Model file for the job. Use its own axes, mm. A direction names the side the tool comes from. Round coordinates to 2 decimals unless told otherwise and drop trailing zeros. Loops run counter-clockwise (first coordinate to the right, second up) from the corner with the lowest first, then second, coordinate; pieces in that order, holes last. Notation, with made-up numbers: (83, -5) -> (100, -5) arc R8 cw to (100, 10) -> close; hole circle Ø3 at (4, 59.25). An arc over 180 degrees is marked (long way). Use a Markdown table: item, result.
from build123d import *

# Parameters (mm, degrees)
SKETCH_R          = 1.5
PAD_DEPTH         = 8
SKETCH001_W       = 18.9
SKETCH001_H       = 25.2
POCKET_DEPTH      = 0.8
SKETCH002_W       = 15
SKETCH002_H       = 2.5
SKETCH002_W_2     = 10.4
POCKET001_DEPTH   = 3
SKETCH003_W       = 6
SKETCH003_H       = 30
PAD001_DEPTH      = 9
SKETCH004_W       = 19.2
SKETCH004_H       = 2
POCKET002_DEPTH   = 2
POCKET003_DEPTH   = 3
PAD002_DEPTH      = 3
PAD002_DEPTH_BACK = 3
PAD003_DEPTH      = 1
CHAMFER_SIZE      = 0.95


with BuildPart() as part:
    # Sketch → Pad (new body)
    with BuildSketch(Plane.XY):
        Polygon((-20.1, 15), (11.9, 15), (30, 3.75), (30, -3.75), (11.9, -15), (-20.1, -15), align=None)
        with Locations((-6.25, 0)):
            Circle(SKETCH_R, mode=Mode.SUBTRACT)
    extrude(amount=-PAD_DEPTH)

    # Sketch001 → Pocket (cut)
    with BuildSketch(Plane.XY):
        Rectangle(SKETCH001_W, SKETCH001_H)
    extrude(amount=-POCKET_DEPTH, mode=Mode.SUBTRACT)

    # Sketch002 (on Face33 of Pad003) → Pocket001 (cut)
    with BuildSketch(Plane.XY.offset(-0.8)):
        with Locations((-0.534042, 8.083783)):
            Rectangle(SKETCH002_W, SKETCH002_H)
        with Locations((2.090713, -8.153236)):
            Rectangle(SKETCH002_W_2, SKETCH002_H)
    extrude(amount=-POCKET001_DEPTH, mode=Mode.SUBTRACT)

    # Sketch003 (on Face4 of Pocket001) → Pad001 (join)
    with BuildSketch(Plane.XY):
        with Locations((-17.1, 0)):
            Rectangle(SKETCH003_W, SKETCH003_H)
    extrude(amount=PAD001_DEPTH)

    # Sketch004 (on Face10 of Pad001) → Pocket002 (cut)
    with BuildSketch(Plane.YZ.offset(-14.1)):
        with Locations((0, 6.14)):
            Rectangle(SKETCH004_W, SKETCH004_H)
    extrude(amount=-POCKET002_DEPTH, mode=Mode.SUBTRACT)

    # Sketch005 → Pocket003 (cut)
    with BuildSketch(Plane(origin=(0, 0, -8), x_dir=(1, 0, 0), z_dir=(0, 0, -1))):
        Polygon((-4.633419, 2.8), (-7.866581, 2.8), (-9.483162, 0), (-7.866581, -2.8), (-4.633419, -2.8), (-3.016838, 0), align=None)
    extrude(amount=-POCKET003_DEPTH, mode=Mode.SUBTRACT)

    # Sketch006 → Pad002 (join, two sides)
    with BuildSketch(Plane.XZ) as pad002_sk:
        Polygon((13.9, 0), (20.9, 5.25), (26.9, 5.25), (26.9, 0), align=None)
    extrude(amount=PAD002_DEPTH)
    extrude(pad002_sk.sketch, amount=-PAD002_DEPTH_BACK)

    # Sketch007 (on Face32 of Pad002) → Pad003 (join)
    with BuildSketch(Plane.XY.offset(5.25)):
        with BuildLine():
            ThreePointArc((24, -1.925), (25.925, 0), (24, 1.925))
            Line((24, 1.925), (23, 1.925))
            Line((23, 1.925), (23, -1.925))
            Line((23, -1.925), (24, -1.925))
        make_face()
    extrude(amount=PAD003_DEPTH)

    # Chamfer
    chamfer_edges = [part.edges().sort_by_distance(p)[0] for p in [
        (23, 0, 6.25),
        (23, -1.925, 5.75),
        (23, 1.925, 5.75),
    ]]
    chamfer(chamfer_edges, length=CHAMFER_SIZE)


solid = part.part
Q1. Band-saw the part on D-D, the plane z = -1.5. Give the cut face in (x, y), plus the area to 3 significant figures.
Results list:
| item | result |
|---|---|
| outline | (-20.1, -15) -> (11.9, -15) -> (30, -3.75) -> (30, 3.75) -> (11.9, 15) -> (-20.1, 15) -> close; hole (-8.03, 6.83) -> (6.97, 6.83) -> (6.97, 9.33) -> (-8.03, 9.33) -> close; hole circle Ø3 at (-6.25, 0); hole (-3.11, -9.4) -> (7.29, -9.4) -> (7.29, -6.9) -> (-3.11, -6.9) -> close |
| area | 1,230 mm² |
Q2. Band-saw the part on C-C, the plane z = 3. Give the cut face in (x, y).
Results list:
| item | result |
|---|---|
| outline | (-20.1, -15) -> (-14.1, -15) -> (-14.1, 15) -> (-20.1, 15) -> close; (17.9, -3) -> (26.9, -3) -> (26.9, 3) -> (17.9, 3) -> close |
Q3. Band-saw the part on A-A, the plane x = -6.25. Give the cut face in (y, z).
Results list:
| item | result |
|---|---|
| outline | (-15, -8) -> (-2.8, -8) -> (-2.8, -5) -> (-1.5, -5) -> (-1.5, -0.8) -> (-12.6, -0.8) -> (-12.6, 0) -> (-15, 0) -> close; (1.5, -5) -> (2.8, -5) -> (2.8, -8) -> (15, -8) -> (15, 0) -> (12.6, 0) -> (12.6, -0.8) -> (9.33, -0.8) -> (9.33, -3.8) -> (6.83, -3.8) -> (6.83, -0.8) -> (1.5, -0.8) -> close |
Q4. Pull direction Y, two halves, no side cores. Call faces 5 (the face through (20.823, 9.454, -3.944)), 6 (the face through (-15, -9.6, 6)), 7 (the face through (-8, -15, -3)), 8 (the face through (13, 0, 0)): released by +Y, released by -Y, zero draft, split by the parting line, or undercut.
Results list:
| item | result |
|---|---|
| face 5 | released by +Y |
| face 6 | undercut |
| face 7 | released by -Y |
| face 8 | zero draft |
Q5. Tool access for faces 1 (the face through (0, 0, -0.8)), 2 (the face through (23.574, -1.549, 5.632)), 3 (the face through (-3.836, 1.42, -6.521)), 4 (the face through (17.35, -0.04, 2.59)): list every direction of +Z, -Z, +X, -X, +Y, -Y with a clear straight run to the whole face (end or side of a thin tool).
Results list:
| item | result |
|---|---|
| face 1 | +Z |
| face 2 | +Z, -Y |
| face 3 | -Z |
| face 4 | +Z, +Y, -Y |
Q6. Drill centre lines: L1, parallel to Y at x = -6.25, z = -1.8; L2, parallel to Y at x = 17, z = 0.25; L3, parallel to Z at x = -8, y = 3. Where is each one in solid material? Low to high. Write a range as from..to.
Results list:
| item | result |
|---|---|
| L1 | y = -15..-1.5, 1.5..6.83, 9.33..15 |
| L2 | y = -3..3 |
| L3 | z = -8..-0.8 |
Q7. Flat gauge pins, fed straight in: pin 1 (1 mm diameter, centred on x = -6.5, y = 1, fed in from -Z); pin 2 (6 mm diameter, centred on x = -6, y = -1, fed in from -Z); pin 3 (2 mm diameter, centred on y = -6, z = 4, fed in from +X); pin 4 (6 mm diameter, centred on x = 17.5, z = 2, fed in from -Y). Where does each tip first touch, or does it go through?
Results list:
| item | result |
|---|---|
| pin 1 | stops at z = -5 |
| pin 2 | stops at z = -8 |
| pin 3 | stops at x = -14.1 |
| pin 4 | stops at y = -12.91 |
Q8. Band-saw the part on B-B, the plane z = -5.75. Give the cut face in (x, y), plus the area to 3 significant figures.
Results list:
| item | result |
|---|---|
| outline | (-20.1, -15) -> (11.9, -15) -> (30, -3.75) -> (30, 3.75) -> (11.9, 15) -> (-20.1, 15) -> close; hole (-9.48, 0) -> (-7.87, -2.8) -> (-4.63, -2.8) -> (-3.02, 0) -> (-4.63, 2.8) -> (-7.87, 2.8) -> close |
| area | 1,270 mm² |
